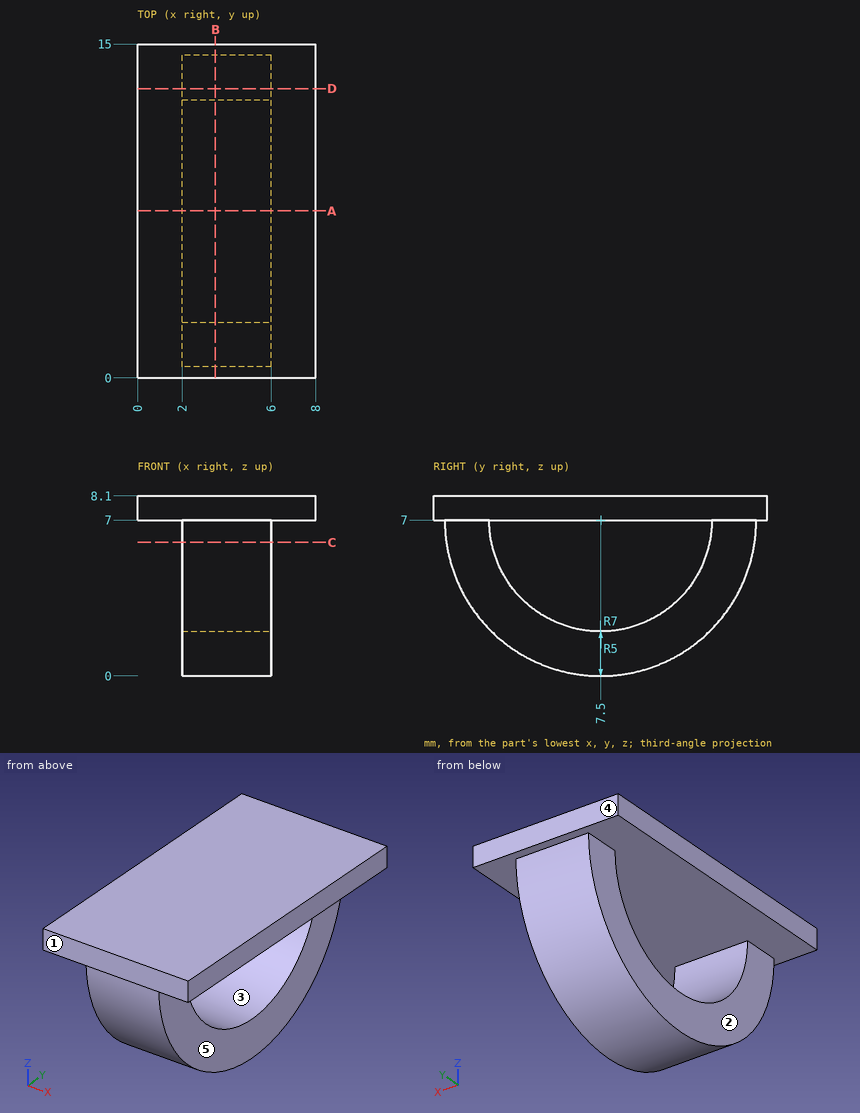
Study the drawing (mm; zero at the part's minimum x, y, z) and answer. A direction names the side the tool comes from. Coordinates: 2 decimals unless noted, no trailing zeros. Write each loop counter-clockwise with the first axis right and the second up, starting at its lowest first coordinate (ties: lowest second). Pieces come first, ordered by that corner, then holes.
Q1. Section A-A, the plane y = 7.5 is taken. Write down the section's boundary in (x, z).
Returned:
outline: (0, 7) - (8, 7) - (8, 8.1) - (0, 8.1) - close; (2, 0) - (6, 0) - (6, 2) - (2, 2) - close
Q2. Section B-B, the plane x = 3.5 is taken. Write down the section's boundary in (y, z), then the cut area to 3 significant figures.
Returned:
outline: (0, 7) - (0.5, 7) arc R7 ccw to (14.5, 7) - (15, 7) - (15, 8.1) - (0, 8.1) - close; hole (2.5, 7) arc R5 ccw to (12.5, 7) - close
area: 54.2 mm2
Q3. The mould has two halves that part along Y. Classify the marked faces 1, 2 and 3: released by +Y, released by -Y, zero draft, split by the parting line, or undercut.
Returned:
face 1: released by -Y
face 2: zero draft
face 3: undercut
Q4. Find the intervals of material crossed by line 1 along Z through (x, y) = (7.25, 8.25); line 2 along X through (y, z) = (3.25, 2); line 3 along Y through (x, z) = (3, 4.25), in increasing order.
Returned:
line 1: z = 7 to 8.1
line 2: x = 2 to 6
line 3: y = 1.06 to 3.32, 11.68 to 13.94
Q5. Given P1, Ø2, axis at x = 1.5, z = 5, coming from the +Y side; P2, Ø3, axis at y = 5, z = 4, coming from the -X side; P3, Ø2, axis at y = 4, z = 4.5, coming from the +X side, each flat-ended and moving along its own axis, determine where each tip first touches the part or whether it passes through.
Returned:
P1: stops at y = 14.41
P2: stops at x = 2
P3: stops at x = 6
Q6. Section C-C, the plane z = 6 is taken. Write down the section's boundary in (x, y).
Returned:
outline: (2, 0.57) - (6, 0.57) - (6, 2.6) - (2, 2.6) - close; (2, 12.4) - (6, 12.4) - (6, 14.43) - (2, 14.43) - close
Q7. Section D-D, the plane y = 13 is taken. Write down the section's boundary in (x, z), then the cut area to 3 significant figures.
Returned:
outline: (0, 7) - (2, 7) - (2, 2.67) - (6, 2.67) - (6, 7) - (8, 7) - (8, 8.1) - (0, 8.1) - close
area: 26.1 mm2
Q8. Which of the six approach directions +Z, -Z, +X, -X, +Y, -Y give full straight-line access (tool end or side, diameter ignored) to the marked faces 4 and 5?
Returned:
face 4: +Z, -Z, +X, -X, +Y
face 5: -Z, +X, +Y, -Y
